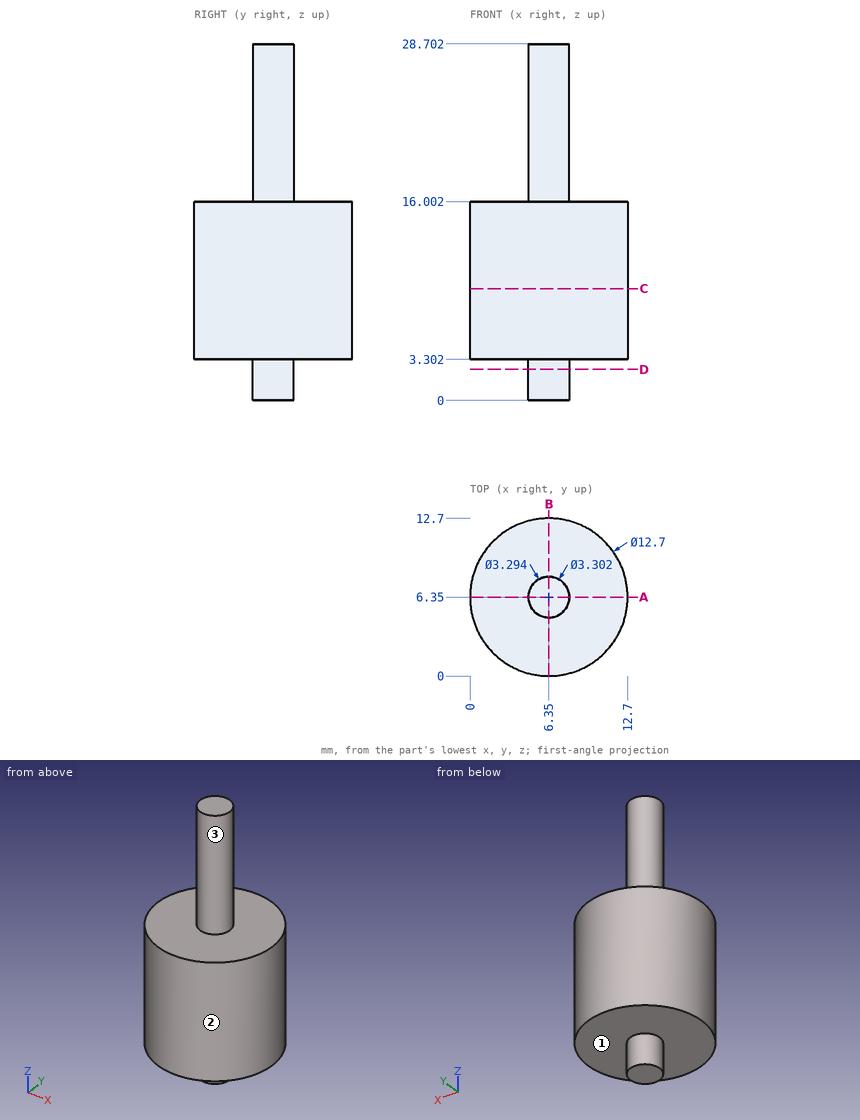
Check sheet for the drawn part. Datum: minimum x, y, z corner. Units: mm. A direction names the side the tool comes from. Give positions to 0.01 mm unless a question says otherwise; leave off trailing zeros. Loops run counter-clockwise (first coordinate to the right, second up) from the corner with the lowest first, then second, coordinate; pieces in that order, holes last. Notation, with made-up numbers: M 78,67.5 L 129,67.5 A13 cw 129,74.5 Z; hole C -9,-37.5 d9. An arc over 180 degrees is marked long. Return JSON: item names as keys, results as strings.
1) Section check C-C, the plane z = 9. Enter the section's corners in (x, y).
Findings:
{"outline": "C 6.35,6.35 d12.7"}
2) Gauge pin test, flat ends, axial feed: P1, Ø5, axis at x = 2.5, z = 19, coming from the -Y side; P2, Ø1.5, axis at x = 8, z = 24, coming from the -Y side; P3, Ø4, axis at x = 4, z = 5.5, coming from the -Y side. Record the tip position at first contact, or that the pin passes through.
Findings:
{"P1": "stops at y = 5.4", "P2": "stops at y = 4.97", "P3": "stops at y = 0.01"}
3) Section check A-A, the plane y = 6.35. Enter the section's corners in (x, z).
Findings:
{"outline": "M 0,3.3 L 4.7,3.3 L 4.7,0 L 8,0 L 8,3.3 L 12.7,3.3 L 12.7,16 L 8,16 L 8,28.7 L 4.7,28.7 L 4.7,16 L 0,16 Z"}
4) Tool access check on the marked faces 1, 2 and 3. Record the directions out of +Z, -Z, +X, -X, +Y, -Y that give a thin tool (end or side, any length) a straight path to the whole face; none if there is none.
Findings:
{"face 1": "-Z", "face 2": "+Z, -Z", "face 3": "+Z"}
5) Section check D-D, the plane z = 2.5. Enter the section's corners in (x, y), and give its area (3 significant figures).
Findings:
{"outline": "C 6.35,6.35 d3.29", "area": "8.52 mm2"}
6) Material ranges on L1, parallel to Z at x = 6.75, y = 3; L2, parallel to X at y = 6.5, z = 13.75; L3, parallel to Y at x = 7, z = 21.5, recorded low to high. Write a range as [from, to].
Findings:
{"L1": "z = [3.3, 16]", "L2": "x = [0, 12.7]", "L3": "y = [4.83, 7.87]"}
